```python
from build123d import *

# Parameters (mm, degrees)
F0_R     = 11.2
F1_DEPTH = 7
F2_R     = 1.5
F3_R     = 1.5


with BuildPart() as f1:
    # F0 (on Top) → F1 (new body)
    with BuildSketch(Plane.XY):
        with BuildLine():
            Line((-13.195308, 26.308456), (-13.195308, -26.457274))
            ThreePointArc((-13.195308, -26.457274), (0.004692, -39.657274), (13.204692, -26.457274))
            Line((13.204692, -26.457274), (13.204692, 26.308456))
            ThreePointArc((13.204692, 26.308456), (0.004692, 39.508456), (-13.195308, 26.308456))
        make_face()
        with Locations((0.004692, -26.457274)):
            Circle(F0_R, mode=Mode.SUBTRACT)
        with Locations((0.004692, 26.308456)):
            Circle(F0_R, mode=Mode.SUBTRACT)
        with Locations((0.004719, -0.073227)):
            Circle(F0_R, mode=Mode.SUBTRACT)
    extrude(amount=F1_DEPTH)

    # F2
    f2_edges = [f1.edges().sort_by_distance(p)[0] for p in [
        (-13.195308, -0.074409, 7),
        (0.004692, 39.508456, 7),
        (13.204692, -0.074409, 7),
        (0.004692, -39.657274, 7),
    ]]
    fillet(f2_edges, radius=F2_R)

    # F3
    f3_edges = [f1.edges().sort_by_distance(p)[0] for p in [
        (13.204692, -0.074409, 0),
        (0.004692, 39.508456, 0),
        (-13.195308, -0.074409, 0),
        (0.004692, -39.657274, 0),
    ]]
    fillet(f3_edges, radius=F3_R)


solid = f1.part
```
Model file for the job. Use its own axes, mm. Give positions to 0.01 mm unless a question says otherwise; leave off trailing zeros. Loops run counter-clockwise (first coordinate to the right, second up) from the corner with the lowest first, then second, coordinate; pieces in that order, holes last. Notation, with made-up numbers: (44.5, -28) - (63.5, -28) arc R34 cw to (63.5, 8) - close; hole circle Ø9 at (-35.75, 6.25). An arc over 180 degrees is marked (long way). One line per item, written item: value. Start each with the question number.
1. Slice it at D-D (y = -21). List the corners of the cut face in (x, z).
2. Slice it at B-B (z = 3.75). List the corners of the cut face in (x, y).
3. Pin check, flat tips, straight feed: pin 1 (1.5 mm diameter, centred on x = -3.5, z = 5.5, fed in from +Y); pin 2 (2 mm diameter, centred on x = -5.5, z = 2.5, fed in from +Y); pin 3 (1.5 mm diameter, centred on y = 30.5, z = 6, fed in from -X). Stop position of each tip, or through.
4. Probe L1, parallel to X at y = 26.5, z = 2; L2, parallel to Y at x = 0.75, z = 6.5; L3, parallel to Y at x = 8.5, z = 3. List the from-to ranges inside material, lowest first. Write a range as from..to.
5. Slice it at A-A (y = 1.5). List the corners of the cut face in (x, z), plus the area to 3 significant figures.
6. Slice it at C-C (x = -1). Give the number of separate pieces and of enclosed holes in the cut face, plus the area to 3 significant figures.
7. Pull direction X, two halves, no side cores. Call faces 1 (the cylindrical face through (-1.453, -15.353, 3.451)), 2 (the flat face through (13.205, 0, 3)), 3 (the flat face through (0.8, 11.4, 7)), 4 (the flat face through (-13.195, 0, 3)): pulls with the +X half, pulls with the -X half, needs draft (parallel to the pull), parting line crosses it, or undercut.
Solution:
1. outline: (-13.2, 1.5) arc R1.5 ccw to (-11.7, 0) - (-9.78, 0) - (-9.78, 7) - (-11.7, 7) arc R1.5 ccw to (-13.2, 5.5) - close; (9.79, 0) - (11.7, 0) arc R1.5 ccw to (13.2, 1.5) - (13.2, 5.5) arc R1.5 ccw to (11.7, 7) - (9.79, 7) - close
2. outline: (-13.2, -26.46) arc R13.2 ccw to (13.2, -26.46) - (13.2, 26.31) arc R13.2 ccw to (-13.2, 26.31) - close; hole circle Ø22.4 at (0, -26.46); hole circle Ø22.4 at (0, -0.07); hole circle Ø22.4 at (0, 26.31)
3. pin 1: stops at y = 39.22
3. pin 2: stops at y = 38.72
3. pin 3: stops at x = -12.71
4. L1: x = -13.19..-11.19, 11.2..13.2
4. L2: y = -39.25..-37.63, -15.28..-11.25, 11.1..15.13, 37.48..39.1
4. L3: y = -36.56..-33.76, -19.16..-7.37, 7.23..19.01, 33.61..36.41
5. outline: (-13.2, 1.5) arc R1.5 ccw to (-11.7, 0) - (-11.08, 0) - (-11.08, 7) - (-11.7, 7) arc R1.5 ccw to (-13.2, 5.5) - close; (11.09, 0) - (11.7, 0) arc R1.5 ccw to (13.2, 1.5) - (13.2, 5.5) arc R1.5 ccw to (11.7, 7) - (11.09, 7) - close
5. area: 27.6 mm^2
6. separate pieces: 4
6. enclosed holes: 0
6. area: 83.2 mm^2
7. face 1: undercut
7. face 2: pulls with the +X half
7. face 3: needs draft
7. face 4: pulls with the -X half
